Work out the finished part from the listing and answer in its coordinate system (mm). A direction names the side the tool comes from. Coordinates: 2 decimals unless noted, no trailing zeros. Order: outer loops, then holes, each group sorted by start corner. A loop starts at its lowest first (then second) coordinate and runs counter-clockwise, first axis right, second up. Notation, with made-up numbers: (-24, 75) - (-20, 75) arc R7 cw to (-20, 79) - close; hole circle Ø8 at (-31.5, 88). An arc over 180 degrees is marked (long way). Answer as a JSON object with one key per item and string values. Group by question number.
1) A tool of negligible diameter and unlimited length cuts with its end or side. For faces 5 (the face through (57.493, 20, 1)), 6 (the face through (1, 19, -47.003)), 7 (the face through (58.607, 31.282, 19.112)), from which of +Z, -Z, +X, -X, +Y, -Y can it reach the whole face along a straight path? Write none if from no direction.
2) Find the intervals of material crossed by line 1 along X through (y, z) = (-0.4, 25.4); line 2 along Z through (x, y) = (11, 23); line 3 along X through (y, z) = (16, 36.5), in increasing order.
3) Section A-A (x = 0) is taken. Give the vertices of the cut face in (y, z).
4) Section C-C (y = 10.5) is taken. Give the vertices of the cut face in (x, z), plus the area to 3 significant figures.
5) The mould has two halves that part along X. Classify faces 1 (the face through (1, -1.13, 1)), 2 (the face through (-59.754, 19, -1)), 3 (the face through (-38.902, 0.016, 25.239)), 4 (the face through (32.67, 0.016, 11.458)): released by +X, released by -X, zero draft, split by the parting line, or undercut.
6) Section B-B (z = 40.5) is taken. Give the vertices of the cut face in (x, y), plus the area to 3 significant figures.
7) Each of these flat-tipped pins is pushed along its axis until it touches: P1, Ø1.8, axis at x = 32.99, z = 9.99, coming from the -Y side; P2, Ø3.5, axis at x = -40.26, z = -25.67, coming from the +Y side. Where does it stop, or does it pass through?
8) Section D-D (x = -48.5) is taken. Give the vertices of the cut face in (y, z).
Autodesk Inventor part; units mm, degrees
ref_plane "YZ Plane" through (0, 0, 0) normal (1, 0, 0) x (0, 1, 0)
ref_plane "XZ Plane" through (0, 0, 0) normal (0, 1, 0) x (-1, 0, 0)
ref_plane "XY Plane" through (0, 0, 0) normal (0, 0, 1) x (1, 0, 0)
sketch "Sketch1" plane through (0, 0, 0) normal (0, 1, 0) x (-1, 0, 0)
  line L0 (-59.7535, -47.0027) -> (59.7535, -47.0027)
  line L1 (59.7535, -47.0027) -> (59.7535, 47.0027)
  line L2 (59.7535, 47.0027) -> (-59.7535, 47.0027)
  line L3 (-59.7535, 47.0027) -> (-59.7535, -47.0027)
  line L4 (-59.7535, -47.0027) -> (59.7535, 47.0027) construction
  line L5 (59.7535, -47.0027) -> (-59.7535, 47.0027) construction
  point P0 (0, 0)
  dimension "d0" = 119.507
  dimension "d1" = 94.0054
extrude "Extrusion1" add sketch "Sketch1" along normal mid plane 2.2606
sketch "Sketch2" plane through (0, 1.1303, 0) normal (0, 1, 0) x (1, 0, 0)
  line L0 (-59.7535, 47.0027) -> (-59.7535, -47.0027)
  line L1 (59.7535, -47.0027) -> (59.7535, 47.0027)
  line L2 (-59.7535, -47.0027) -> (59.7535, -47.0027)
  line L3 (59.7535, -47.0027) -> (59.7535, 47.0027)
  line L4 (59.7535, 47.0027) -> (-59.7535, 47.0027)
  line L5 (-59.7535, 47.0027) -> (-59.7535, -47.0027)
  line L6 (57.4929, -44.7421) -> (-57.4929, 44.7421) construction
  line L7 (-57.4929, -44.7421) -> (57.4929, 44.7421) construction
  line L8 (-59.7535, -47.0027) -> (59.7535, -47.0027)
  line L9 (-59.7535, -47.0027) -> (-50.7619, -47.0027)
  line L10 (-59.7535, -38.0111) -> (-59.7535, -47.0027)
  line L11 (-59.7535, 47.0027) -> (-50.7619, 47.0027)
  line L12 (-59.7535, 38.0111) -> (-59.7535, 47.0027)
  line L13 (59.7535, 47.0027) -> (-59.7535, 47.0027)
  line L14 (59.7535, 47.0027) -> (50.7619, 47.0027)
  line L15 (59.7535, 38.0111) -> (59.7535, 47.0027)
  line L16 (59.7535, -47.0027) -> (50.7619, -47.0027)
  line L17 (59.7535, -38.0111) -> (59.7535, -47.0027)
  line L18 (-50.7619, -44.7421) -> (-50.7619, -38.0111)
  line L19 (-50.7619, -38.0111) -> (-57.4929, -38.0111)
  line L20 (-57.4929, 38.0111) -> (-50.7619, 38.0111)
  line L21 (-50.7619, 38.0111) -> (-50.7619, 44.7421)
  line L22 (50.7619, 38.0111) -> (57.4929, 38.0111)
  line L23 (50.7619, 44.7421) -> (50.7619, 38.0111)
  line L24 (57.4929, -38.0111) -> (50.7619, -38.0111)
  line L25 (50.7619, -38.0111) -> (50.7619, -44.7421)
  line L26 (-50.7619, -44.7421) -> (50.7619, -44.7421)
  line L27 (57.4929, -38.0111) -> (57.4929, 38.0111)
  line L28 (50.7619, 44.7421) -> (-50.7619, 44.7421)
  line L29 (-57.4929, 38.0111) -> (-57.4929, -38.0111)
  point P0 (0, 0)
  dimension "d4" = 114.9858
  dimension "d5" = 89.4842
  dimension "d6" = 8.9916
  dimension "d7" = 8.9916
  dimension "d10" = 8.9916
  dimension "d11" = 8.9916
extrude "Extrusion2" add sketch "Sketch2" along normal blind 38.1
sketch "Sketch3" plane through (0, 1.1303, 0) normal (0, 1, 0) x (1, 0, 0)
  circle A0 centre (0, -25.4) radius 2.0828
  circle A1 centre (0, 25.4) radius 2.0828
  point P0 (0, 0)
  dimension "d18" = 4.1656
  dimension "d19" = 4.1656
extrude "Extrusion3" cut sketch "Sketch3" against normal through all
sketch "Sketch4" plane through (0, 1.1303, 0) normal (0, 1, 0) x (1, 0, 0)
  line L0 (43.434, -28.8417) -> (-43.434, 28.8417) construction
  line L1 (-43.434, -28.8417) -> (43.434, 28.8417) construction
  line L2 (32.9946, -9.9949) -> (-32.9946, 9.9949) construction
  line L3 (-32.9946, -9.9949) -> (32.9946, 9.9949) construction
  circle A0 centre (-40.259, -25.6667) radius 1.4224
  circle A1 centre (-40.259, 25.6667) radius 1.4224
  circle A2 centre (18.034, -25.6667) radius 1.4224
  circle A3 centre (18.034, 25.6667) radius 1.4224
  circle A4 centre (-32.9946, -9.9949) radius 1.4986
  circle A5 centre (-32.9946, 9.9949) radius 1.4986
  circle A6 centre (32.9946, 9.9949) radius 1.4986
  circle A7 centre (32.9946, -9.9949) radius 1.4986
  point P0 (0, 0)
  point P1 (0, 0)
  dimension "d22" = 86.868
  dimension "d23" = 57.6834
  dimension "d25" = 19.9898
  dimension "d30" = 2.8448
  dimension "d31" = 2.8448
  dimension "d36" = 2.8448
  dimension "d37" = 2.8448
  dimension "d38" = 2.9972
  dimension "d39" = 2.9972
  dimension "d40" = 2.9972
  dimension "d41" = 2.9972
extrude "Extrusion4" cut sketch "Sketch4" against normal through all
sketch "Sketch6" plane through (57.4929, 1.1303, -38.0111) normal (-1, 0, 0) x (0, 0, 1)
  circle A0 centre (53.7096, 24.7973) radius 6.35
  point P0 (38.0111, -1.1303)
  dimension "d44" = 12.7
extrude "Extrusion5" cut sketch "Sketch6" against normal through all
sketch "Sketch7" plane through (-50.7619, 1.1303, -44.7421) normal (0, 0, 1) x (1, 0, 0)
  line L0 (12.3731, 32.369) -> (63.1731, 32.369)
  line L1 (63.1731, 32.369) -> (63.1731, 27.0954)
  line L2 (63.1731, 27.0954) -> (12.3731, 27.0954)
  line L3 (12.3731, 27.0954) -> (12.3731, 32.369)
  point P0 (50.7619, -1.1303)
  dimension "d47" = 50.8
extrude "Extrusion6" cut sketch "Sketch7" against normal through all
properties part number "546-1590BBS-Pi"
Report:
{
 "1": {"face 5": "+Y", "face 6": "-Z, +X, -X, +Y, -Y", "face 7": "+X"},
 "2": {"line 1": "x = -59.75 to -41.66, -38.86 to -2.08, 2.08 to 16.64, 19.43 to 59.75", "line 2": "z = -47 to -44.74, 44.74 to 47", "line 3": "x = -59.75 to -57.49, 57.49 to 59.75"},
 "3": {"outline": "(-1.13, -47) - (28.23, -47) - (28.23, -44.74) - (1.13, -44.74) - (1.13, -27.48) - (-1.13, -27.48) - close; (-1.13, -23.32) - (1.13, -23.32) - (1.13, 23.32) - (-1.13, 23.32) - close; (-1.13, 27.48) - (1.13, 27.48) - (1.13, 44.74) - (39.23, 44.74) - (39.23, 47) - (-1.13, 47) - close; (33.5, -47) - (39.23, -47) - (39.23, -44.74) - (33.5, -44.74) - close"},
 "4": {"outline": "(-59.75, -47) - (59.75, -47) - (59.75, 47) - (-59.75, 47) - close; hole (-57.49, -38.01) - (-50.76, -38.01) - (-50.76, -44.74) - (50.76, -44.74) - (50.76, -38.01) - (57.49, -38.01) - (57.49, 38.01) - (50.76, 38.01) - (50.76, 44.74) - (-50.76, 44.74) - (-50.76, 38.01) - (-57.49, 38.01) - close", "area": "1,130 mm²"},
 "5": {"face 1": "zero draft", "face 2": "released by -X", "face 3": "undercut", "face 4": "undercut"},
 "6": {"outline": "(-59.75, -1.13) - (59.75, -1.13) - (59.75, 39.23) - (50.76, 39.23) - (50.76, 1.13) - (-50.76, 1.13) - (-50.76, 39.23) - (-59.75, 39.23) - close", "area": "955 mm²"},
 "7": {"P1": "passes through", "P2": "stops at y = 1.13"},
 "8": {"outline": "(-1.13, -47) - (39.23, -47) - (39.23, -44.74) - (1.13, -44.74) - (1.13, 44.74) - (39.23, 44.74) - (39.23, 47) - (-1.13, 47) - close"}
}
